Can you work these out from the model? Positions are in its coordinate system, mm. Face numbers are marked on the shaded views. A direction names the side the tool comes from. Round coordinates to 2 decimals unless told otherwise and drop trailing zeros. Order: outer loops, then holes, each group sorted by start corner. A loop starts at its lowest first (then second) coordinate and runs counter-clockwise, first axis right, second up. Notation, with made-up numbers: (17, 55) -> (59, 55) arc R32 cw to (59, 84) -> close; hole circle Ø8 at (7.5, 25.25). An arc over 180 degrees is marked (long way). One line per item, written item: value.
Autodesk Fusion 360 part; units mm, degrees
sketch "Sketch1" plane through (0, 0, 0) normal (0, 1, 0) x (1, 0, 0)
  line L0 (-0.3317, -1.9864) -> (56.6183, -1.9864)
  line L1 (56.6183, -1.9864) -> (56.6183, -51.9564)
  line L2 (56.6183, -51.9564) -> (-0.3317, -51.9564)
  line L3 (-0.3317, -51.9564) -> (-0.3317, -1.9864)
  line L4 (-5.3317, 3.0136) -> (61.6183, 3.0136)
  line L5 (61.6183, 3.0136) -> (61.6183, -56.9564)
  line L6 (61.6183, -56.9564) -> (-5.3317, -56.9564)
  line L7 (-5.3317, -56.9564) -> (-5.3317, 3.0136)
  circle A0 centre (59.1183, -54.4564) radius 1.5
  circle A1 centre (-2.8317, -54.4564) radius 1.5
  circle A2 centre (-2.8317, 0.5136) radius 1.5
  circle A3 centre (59.1183, 0.5136) radius 1.5
  circle A4 centre (-2.8317, -54.4564) radius 2
  circle A5 centre (59.1183, -54.4564) radius 2
  circle A6 centre (59.1183, 0.5136) radius 2
  circle A7 centre (-2.8317, 0.5136) radius 2
  dimension "d2" = 49.97
  dimension "d3" = 66.95
  dimension "d4" = 59.97
  dimension "d5" = 5
  dimension "d6" = 5
  dimension "d7" = 3
  dimension "d8" = 3
  dimension "d9" = 3
  dimension "d10" = 3
  dimension "d11" = 2.5
  dimension "d12" = 2.5
  dimension "d13" = 2.5
  dimension "d14" = 2.5
  dimension "d15" = 2.5
  dimension "d16" = 2.5
  dimension "d17" = 2.5
  dimension "d18" = 2.5
  dimension "d19" = 4
  dimension "d20" = 4
  dimension "d21" = 4
  dimension "d22" = 4
extrude "Extrude1" add sketch "Sketch1" along normal blind 3 contours L0 L1 L2 L3
extrude "Extrude2" add sketch "Sketch1" along normal blind 14 contours L4 L5 L6 L7 | A4 | A5 | A6 | A7
extrude "Extrude3" add sketch "Sketch1" along normal blind 13 contours A0 | A1 | A2 | A3
sketch "Sketch2" plane through (0, 14, 0) normal (0, 1, 0) x (-1, 0, 0)
  circle A0 centre (2.8317, 54.4564) radius 1.5
  circle A1 centre (-59.1183, -0.5136) radius 1.5
  circle A2 centre (-59.1183, 54.4564) radius 1.5
  line L0 (-56.6183, 51.9564) -> (0.3317, 51.9564)
  line L1 (0.3317, 51.9564) -> (0.3317, 1.9864)
  line L2 (0.3317, 1.9864) -> (-56.6183, 1.9864)
  line L3 (-56.6183, 1.9864) -> (-56.6183, 51.9564)
  circle A3 centre (2.8317, -0.5136) radius 1.5
  line L4 (5.3317, 56.9564) -> (-61.6183, 56.9564)
  line L5 (-61.6183, 56.9564) -> (-61.6183, -3.0136)
  line L6 (-61.6183, -3.0136) -> (5.3317, -3.0136)
  line L7 (5.3317, -3.0136) -> (5.3317, 56.9564)
  line L8 (0.3317, 1.9864) -> (-30.6683, 1.9864)
  line L9 (-30.6683, 1.9864) -> (-30.6683, -3.0136)
  line L10 (-30.6683, -3.0136) -> (0.3317, -3.0136)
  line L11 (0.3317, -3.0136) -> (0.3317, 1.9864)
  line L12 (0.3317, 51.9564) -> (-30.6683, 51.9564)
  line L13 (-30.6683, 51.9564) -> (-30.6683, 56.9564)
  line L14 (-30.6683, 56.9564) -> (0.3317, 56.9564)
  line L15 (0.3317, 56.9564) -> (0.3317, 51.9564)
  dimension "d29" = 31
  dimension "d30" = 31
extrude "Extrude4" cut sketch "Sketch2" against normal blind 11 contours L0 L4 L12 L13 L14 L15
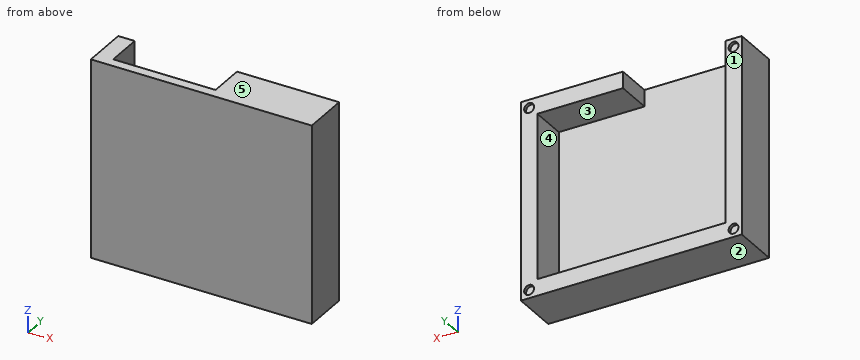
Q1. Please list where these lines run through material, in increasing order: line 1 along X through (y, z) = (6, 44.5); line 2 along Z through (x, y) = (52, 4); line 3 along Y through (x, z) = (38, 37).
Answers below:
line 1: -5.33 to -0.33, 56.62 to 61.62
line 2: -3.01 to 1.99, 51.96 to 56.96
line 3: 0 to 3
Q2. On a 3-axis mill with a long thin cutter (end or side, diameter ignored), from which of +Z, -Z, +X, -X, +Y, -Y can I reach the whole of each face in a straight line? I mean the marked faces 4 and 5. Say none if no direction works.
Answers below:
face 4: +Y
face 5: +Z, +X, -X, +Y, -Y
Q3. Will these pins go through, and if not, where does the flat tip stop? pin 1 Ø10 at (x, z) = (41, 13) entering from +Y; pin 2 Ø1.5 at (x, z) = (59.5, -1) entering from +Y.
Answers below:
pin 1: y = 3
pin 2: y = 13
Q4. We'd pull the mould along Z, two halves only. Please class the marked faces 1, 2 and 3: released by +Z, released by -Z, zero draft, split by the parting line, or undercut.
Answers below:
face 1: zero draft
face 2: released by -Z
face 3: undercut
Q5. I want a section at B-B on y = 10. List the corners of the cut face in (x, z) for me.
Answers below:
outline: (-5.33, -3.01) -> (61.62, -3.01) -> (61.62, 56.96) -> (30.67, 56.96) -> (30.67, 51.96) -> (56.62, 51.96) -> (56.62, 1.99) -> (-0.33, 1.99) -> (-0.33, 56.96) -> (-5.33, 56.96) -> close
Q6. I want a section at C-C on z = 13. List the corners of the cut face in (x, y) for me, plus the area to 3 significant figures.
Answers below:
outline: (-5.33, 0) -> (61.62, 0) -> (61.62, 14) -> (56.62, 14) -> (56.62, 3) -> (-0.33, 3) -> (-0.33, 14) -> (-5.33, 14) -> close
area: 311 mm^2
Q7. I want a section at A-A on x = 31.5. List the corners of the cut face in (y, z) for me.
Answers below:
outline: (0, -3.01) -> (14, -3.01) -> (14, 1.99) -> (3, 1.99) -> (3, 51.96) -> (14, 51.96) -> (14, 56.96) -> (0, 56.96) -> close
